The listing builds one solid part. Answer for the finished solid, in the listing's coordinates (mm). Face numbers are marked on the shaded views. A direction names the side the tool comes from. Give positions to 0.01 mm unless a question says otherwise; leave off trailing zeros. Order: outer loops, then holes, each group sorted by start corner. A loop starts at its lowest first (then second) coordinate and runs counter-clockwise, first axis right, second up.
```python
from build123d import *

# Parameters (mm, degrees)
BOSS_EXTRUDE1_DEPTH       = 50
SKETCH2_W                 = 15
SKETCH2_H                 = 12
SKETCH2_W_2               = 20
CUT_EXTRUDE1_DEPTH        = 50
CUT_EXTRUDE2_DEPTH        = 50
F_5_0MM_DOWEL_HOLE1_D     = 5
F_5_0MM_DOWEL_HOLE1_DEPTH = 10
F_5_0MM_DOWEL_HOLE1_TIP   = 1.502151548
SKETCH7_R                 = 2.25
CUT_EXTRUDE3_DEPTH        = 10


with BuildPart() as part:
    # Sketch1 → Boss-Extrude1 (new body)
    with BuildSketch(Plane.XY):
        Polygon((-2, -1), (5, -1), (5, 13), (-5, 13), (-5, -13), (5, -13), (5, -11), (-2, -11), align=None)
    extrude(amount=BOSS_EXTRUDE1_DEPTH)

    # Sketch2 → Cut-Extrude1 (cut)
    with BuildSketch(Plane(origin=(5, 0, 0), x_dir=(0, 0, -1), z_dir=(1, 0, 0))):
        with Locations((-42.5, 7)):
            Rectangle(SKETCH2_W, SKETCH2_H)
        with Locations((-10, 7)):
            Rectangle(SKETCH2_W_2, SKETCH2_H)
    extrude(amount=-CUT_EXTRUDE1_DEPTH, mode=Mode.SUBTRACT)

    # Sketch3 → Cut-Extrude2 (cut)
    with BuildSketch(Plane(origin=(-2, 0, 0), x_dir=(0, 0, -1), z_dir=(1, 0, 0))):
        with BuildLine():
            Line((-41, -3), (-9, -3))
            ThreePointArc((-9, -3), (-6, -6), (-9, -9))
            Line((-9, -9), (-41, -9))
            ThreePointArc((-41, -9), (-44, -6), (-41, -3))
        make_face()
    extrude(amount=-CUT_EXTRUDE2_DEPTH, mode=Mode.SUBTRACT)

    # Ø5.0mm Dowel Hole1
    with Locations(Plane(origin=(0, 13, 0), x_dir=(1, 0, 0), z_dir=(0, 1, 0))):
        with Locations((0, -25)):
            Hole(F_5_0MM_DOWEL_HOLE1_D / 2, depth=F_5_0MM_DOWEL_HOLE1_DEPTH)
            with Locations((0, 0, -(F_5_0MM_DOWEL_HOLE1_DEPTH + F_5_0MM_DOWEL_HOLE1_TIP / 2))):  # 118° drill point
                Cone(0, F_5_0MM_DOWEL_HOLE1_D / 2, F_5_0MM_DOWEL_HOLE1_TIP, mode=Mode.SUBTRACT)

    # Sketch7 → Cut-Extrude3 (cut)
    with BuildSketch(Plane.XY.offset(35)):
        with Locations((0, 7)):
            Circle(SKETCH7_R)
    extrude(amount=-CUT_EXTRUDE3_DEPTH, mode=Mode.SUBTRACT)


solid = part.part
```
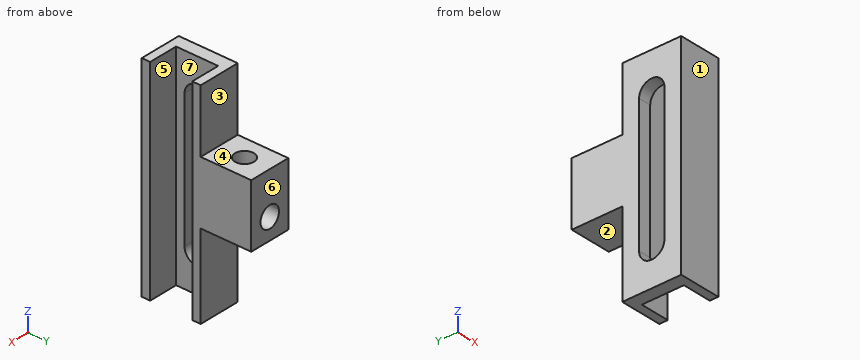
1) Given P1, Ø1, axis at x = -3.5, z = 7.5, coming from the +Y side; P2, Ø6, axis at x = -2.5, y = 8, coming from the +Z side; P3, Ø3.5, axis at x = 0, y = 7, coming from the +Z side, each flat-ended and moving along its own axis, determine where each tip first touches the part or whether it passes through.
Geometry says:
P1: stops at y = 1
P2: stops at z = 35
P3: stops at z = 23.21
2) Find section D-D (x = -3.75). Write down the section's boundary in (y, z), then the cut area to 3 significant figures.
Geometry says:
outline: (-13, 0) - (1, 0) - (1, 20) - (13, 20) - (13, 35) - (1, 35) - (1, 50) - (-13, 50) - close; hole (-9, 9) arc R3 ccw to (-3, 9) - (-3, 41) arc R3 ccw to (-9, 41) - close
area: 660 mm2
3) For a pull along Y with two mould halves and no side action, classify the marked faces 4, 5, 6 and 7 as +Y half, -Y half, draft (parallel to the pull), parting line (faces both ways), or undercut.
Geometry says:
face 4: draft
face 5: undercut
face 6: +Y half
face 7: undercut
4) Find section B-B (x = 4). Write down the section's boundary in (y, z), then the cut area to 3 significant figures.
Geometry says:
outline: (-13, 0) - (-11, 0) - (-11, 50) - (-13, 50) - close; (-1, 0) - (1, 0) - (1, 20) - (13, 20) - (13, 35) - (1, 35) - (1, 50) - (-1, 50) - close
area: 380 mm2
5) A tool of negligible diameter and unlimited length cuts with its end or side. For the marked faces 1, 2 and 3, from which of +Z, -Z, +X, -X, +Y, -Y can it reach the whole face along a straight path? Write none if from no direction.
Geometry says:
face 1: +Z, -Z, +X, -X, -Y
face 2: -Z, +X, -X, +Y
face 3: +Z, +X, -X, +Y
6) Find section A-A (z = 33). Write down the section's boundary in (x, y), then the cut area to 3 significant figures.
Geometry says:
outline: (-5, -13) - (5, -13) - (5, -11) - (-2, -11) - (-2, -9) - (-5, -9) - close; (-5, -3) - (-2, -3) - (-2, -1) - (5, -1) - (5, 13) - (-5, 13) - close; hole circle Ø4.5 at (0, 7)
area: 156 mm2
7) Straight lines are drawn through the part: probe 1 along Y at (x, z) = (0, 30); probe 2 along Y at (x, z) = (-2.5, 41); probe 3 along Y at (x, z) = (-3.5, 21.5). For each, find the intervals that lie inside material, in ascending order.
Geometry says:
probe 1: y = -13 to -11, -1 to 4.75, 9.25 to 13
probe 2: y = -13 to -9, -3 to 1
probe 3: y = -13 to -9, -3 to 13
8) Find section C-C (y = -3.5). Write down the section's boundary in (x, z), then the cut area to 4 significant figures.
Geometry says:
outline: (-5, 0) - (-2, 0) - (-2, 7.34) - (-5, 7.34) - close; (-5, 42.66) - (-2, 42.66) - (-2, 50) - (-5, 50) - close
area: 44.05 mm2
